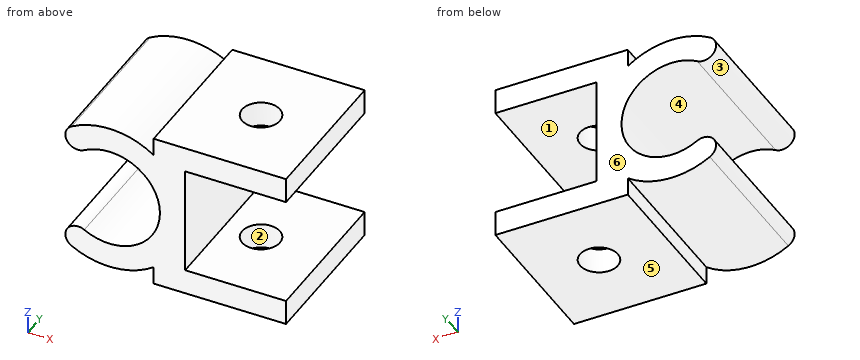
Autodesk Inventor part; units mm, degrees
ref_plane "YZ Plane" through (0, 0, 0) normal (1, 0, 0) x (0, 1, 0)
ref_plane "XZ Plane" through (0, 0, 0) normal (0, 1, 0) x (-1, 0, 0)
ref_plane "XY Plane" through (0, 0, 0) normal (0, 0, 1) x (1, 0, 0)
sketch "Sketch1" plane through (0, 0, 0) normal (0, 1, 0) x (-1, 0, 0)
  line L0 (6.5, 6.3) -> (-4, 6.3)
  line L1 (-4, -6.3) -> (6.5, -6.3)
  line L2 (-4, 4.3) -> (4, 4.3)
  line L3 (4, 4.3) -> (4, -4.3)
  line L4 (4, -4.3) -> (-4, -4.3)
  arc A0 (12, 3.4641) -> (12, -3.4641) centre (10, 0) ccw
  line L5 (6.5, -6.3) -> (6.5, -4.8734)
  line L6 (6.5, 4.8734) -> (6.5, 6.3)
  line L7 (-4, 6.3) -> (-4, 4.3)
  line L8 (-4, -4.3) -> (-4, -6.3)
  arc A1 (12, 3.4641) -> (13, 5.1962) centre (12.5, 4.3301) ccw
  arc A2 (13, -5.1962) -> (12, -3.4641) centre (12.5, -4.3301) ccw
  arc A3 (6.5, -4.8734) -> (13, -5.1962) centre (10, 0) ccw
  arc A4 (13, 5.1962) -> (6.5, 4.8734) centre (10, 0) ccw
  point P0 (0, 0)
  point P1 (4, 0)
  point P2 (-6.8446, 0)
  point P3 (-6.8446, 0)
  point P4 (0, 4.3)
  point P5 (0, -4.3)
  dimension "d1" = 8
  dimension "d2" = 2.5
  dimension "d3" = 8.6
  dimension "d4" = 2
  dimension "d5" = 6
  dimension "d6" = 2.5
  dimension "d7" = 2.5
  dimension "d8" = 6
  dimension "d9" = 6
  dimension "d10" = 8
extrude "Extrusion1" add sketch "Sketch1" along normal blind 12
sketch "Sketch2" plane through (-6.5, 0, 6.3) normal (0, 0, 1) x (1, 0, 0)
  circle A0 centre (5.4, 6) radius 1.5
  line L0 (2.5, 0) -> (2.5, 12)
  point P0 (6.5, 0)
  dimension "d13" = 2.9
  dimension "d14" = 6
  dimension "d15" = 3
extrude "Extrusion2" cut sketch "Sketch2" against normal blind 65.75
properties part number "2mm_3mm Weight Clamp"
Input: part model. Units: mm. Frame: model coordinates. Face numbers are marked on the shaded views. A direction names the side the tool comes from. Give positions to 0.01 mm unless a question says otherwise; leave off trailing zeros. Write each loop counter-clockwise with the first axis right and the second up, starting at its lowest first coordinate (ties: lowest second). Pieces come first, ordered by that corner, then holes.
Q1. Section D-D, the plane z = 3.75. Output: boundary loops of the cut face in (x, y), plus the area to 3 significant figures.
Q2. Pull-direction query (Z, two-part tool) for the marked faces 3, 4, 5 and 6; classes: pulls with the +Z half, pulls with the -Z half, needs draft (parallel to the pull), parting line crosses it, or undercut.
Q3. First-contact query: P1, Ø2.5, axis at x = 0, y = 6, coming from the -Z side; P2, Ø4.5, axis at y = 8, z = 2, coming from the +X side. Flat tips, straight axial feed; report the tip coordinate or a pass-through.
Q4. Set-up query: the marked faces 1 and 2. Return all of +Z, -Z, +X, -X, +Y, -Y with unobstructed straight access to the full face (end or side cutting, diameter ignored); none if empty.
Q5. Section C-C, the plane y = 5.5. Output: boundary loops of the cut face in (x, z).
Q6. Section B-B, the plane x = -1.1. Output: boundary loops of the cut face in (y, z), plus the area to 3 significant figures.
Q7. Section A-A, the plane x = -10. Output: boundary loops of the cut face in (y, z).
Q8. Material intervals for probe 1 along Y at (x, z) = (-1.1, 5.75); probe 2 along Z at (x, y) = (-2.5, 1.25); probe 3 along X at (y, z) = (4, 5), sorted ascending.
Filled in:
1. outline: (-13.31, 0) - (-11.39, 0) - (-11.39, 12) - (-13.31, 12) - close; (-8.61, 0) - (-4, 0) - (-4, 12) - (-8.61, 12) - close
1. area: 78.4 mm2
2. face 3: undercut
2. face 4: undercut
2. face 5: pulls with the -Z half
2. face 6: needs draft
3. P1: stops at z = -6.3
3. P2: stops at x = -4
4. face 1: +X, +Y, -Y
4. face 2: +Z, -Z
5. outline: (-13, -5.2) arc R6 ccw to (-6.5, -4.87) - (-6.5, -6.3) - (-2.51, -6.3) - (-2.51, -4.3) - (-4, -4.3) - (-4, 4.3) - (-2.51, 4.3) - (-2.51, 6.3) - (-6.5, 6.3) - (-6.5, 4.87) arc R6 ccw to (-13, 5.2) arc R1 ccw to (-12, 3.46) arc R4 cw (long way) to (-12, -3.46) arc R1 ccw to start; (0.31, -6.3) - (4, -6.3) - (4, -4.3) - (0.31, -4.3) - close; (0.31, 4.3) - (4, 4.3) - (4, 6.3) - (0.31, 6.3) - close
6. outline: (0, -6.3) - (4.5, -6.3) - (4.5, -4.3) - (0, -4.3) - close; (0, 4.3) - (4.5, 4.3) - (4.5, 6.3) - (0, 6.3) - close; (7.5, -6.3) - (12, -6.3) - (12, -4.3) - (7.5, -4.3) - close; (7.5, 4.3) - (12, 4.3) - (12, 6.3) - (7.5, 6.3) - close
6. area: 36.0 mm2
7. outline: (0, -6) - (12, -6) - (12, -4) - (0, -4) - close; (0, 4) - (12, 4) - (12, 6) - (0, 6) - close
8. probe 1: y = 0 to 4.5, 7.5 to 12
8. probe 2: z = -6.3 to -4.3, 4.3 to 6.3
8. probe 3: x = -13.24 to -6.68, -6.5 to 4
